Autodesk Inventor part; units mm, degrees
ref_plane "YZ Plane" through (0, 0, 0) normal (1, 0, 0) x (0, 1, 0)
ref_plane "XZ Plane" through (0, 0, 0) normal (0, 1, 0) x (-1, 0, 0)
sketch "スケッチ1" plane through (0, 0, 0) normal (0, 1, 0) x (-1, 0, 0)
  circle A0 centre (0, 0) radius 9
  dimension "d0" = 18
extrude "押し出し1" add sketch "スケッチ1" along normal blind 40
sketch "スケッチ2" plane through (0, 0, 0) normal (0, -1, 0) x (1, 0, 0)
  circle A0 centre (0, 0) radius 5.2
  dimension "d4" = 10.4
hole "穴1" at (0, 0, 0) direction (0, 1, 0) diameter 10.4 depth 35
ref_plane "作業平面1" through (0, 0, 9) normal (0, 0, 1) x (1, 0, 0)
sketch "スケッチ3" plane through (0, 0, 9) normal (0, 0, 1) x (1, 0, 0)
  point P0 (0, 0)
  point P1 (0, 7)
hole "穴2" at (0, 7, 9) direction (0, 0, -1) diameter 3 depth 6
ref_plane "作業平面4" through (0, 40, 0) normal (0, 1, 0) x (1, 0, 0)
sketch "スケッチ5" plane through (0, 40, 0) normal (0, 1, 0) x (1, 0, 0)
  circle A0 centre (0, 0) radius 9
  dimension "d41" = 18
extrude "押し出し2" add sketch "スケッチ5" along normal blind 15
ref_plane "作業平面5" through (0, 55, 0) normal (0, 1, 0) x (1, 0, 0)
sketch "スケッチ6" plane through (0, 55, 0) normal (0, 1, 0) x (1, 0, 0)
  circle A0 centre (0, 0) radius 2.6
  dimension "d23" = 5.2
hole "穴3" at (0, 55, 0) direction (0, -1, 0) diameter 5.2 depth 14
sketch "スケッチ7" plane through (0, 0, 9) normal (0, 0, 1) x (1, 0, 0)
  circle A0 centre (0, 48) radius 1.5
  line L0 (9, 55) -> (-9, 55)
  point P0 (0, 0)
  dimension "d31" = 3
  dimension "d42" = 7
hole "穴4" at (0, 48, 9) direction (0, 0, -1) diameter 3 depth 8
ref_plane "作業平面7" through (0, 41, 0) normal (0, 1, 0) x (1, 0, 0)
ref_plane "作業平面8" through (0, 35, 0) normal (0, -1, 0) x (1, 0, 0)
equation "\"d5\" = d4"
properties part number "joint_3D プリント"
Input: part model. Units: mm. Frame: model coordinates. A direction names the side the tool comes from. Give positions to 0.01 mm unless a question says otherwise; leave off trailing zeros. Order: outer loops, then holes, each group sorted by start corner. A loop starts at its lowest first (then second) coordinate and runs counter-clockwise, first axis right, second up.
1. Pin query (flat end, axial travel): pin 1 Ø2 at (x, y) = (-1.5, 30) entering from +Z; pin 2 Ø3 at (x, z) = (0, 0) entering from +Y; pin 3 Ø8 at (x, y) = (-6.5, 47) entering from -Z. Return the tip coordinate at first contact, or that it passes through.
Computed:
pin 1: stops at z = 8.99
pin 2: stops at y = 41
pin 3: stops at z = -8.65
2. Cut plane A-A (x = 0). Return loops of the section in (y, z).
Computed:
outline: (0, -9) - (55, -9) - (55, -2.6) - (41, -2.6) - (41, 2.6) - (46.5, 2.6) - (46.5, 9) - (8.5, 9) - (8.5, 5.2) - (35, 5.2) - (35, -5.2) - (0, -5.2) - close; (0, 5.2) - (5.5, 5.2) - (5.5, 9) - (0, 9) - close; (49.5, 2.6) - (55, 2.6) - (55, 9) - (49.5, 9) - close
3. Set-up query: faces 5 (the face through (-0.59, 27.12, -8.98)), 6 (the face through (0, 35, 0)), 7 (the face through (-0.1, 47.9, -2.6)). Return all of +Z, -Z, +X, -X, +Y, -Y with unobstructed straight access to the full face (end or side cutting, diameter ignored); none if empty.
Computed:
face 5: +Y, -Y
face 6: -Y
face 7: +Y
4. Cut plane B-B (y = 51). Return loops of the section in (x, z), and give its area (3 significant figures).
Computed:
outline: circle Ø18 at (0, 0); hole circle Ø5.2 at (0, 0)
area: 233 mm2
5. Cut plane C-C (z = -4.5). Return loops of the section in (x, y), and give its area (3 significant figures).
Computed:
outline: (-7.79, 0) - (-2.61, 0) - (-2.61, 35) - (2.61, 35) - (2.61, 0) - (7.79, 0) - (7.79, 55) - (-7.79, 55) - close
area: 675 mm2
6. Draft query along Y for faces 1 (the face through (0, 41, 0)), 2 (the face through (1.464, 7.325, 6.961)), 3 (the face through (-0.07, 49.5, 5.51)), 4 (the face through (-4, 0, -4)). Return one class per face: released by +Y, released by -Y, zero draft, split by the parting line, or undercut.
Computed:
face 1: released by +Y
face 2: undercut
face 3: undercut
face 4: released by -Y
7. Line query: probe 1 along Y at (x, z) = (0, 8); probe 2 along Z at (x, y) = (0, 27.5); probe 3 along X at (y, z) = (46, 0). Output: solid intervals per line, ascending.
Computed:
probe 1: y = 0 to 5.5, 8.5 to 46.5, 49.5 to 55
probe 2: z = -9 to -5.2, 5.2 to 9
probe 3: x = -9 to -2.6, 2.6 to 9
8. Cut plane D-D (z = 3.25). Return loops of the section in (x, y).
Computed:
outline: (-8.39, 0) - (-4.06, 0) - (-4.06, 35) - (4.06, 35) - (4.06, 0) - (8.39, 0) - (8.39, 55) - (-8.39, 55) - close; hole circle Ø3 at (0, 48)
